```python
from build123d import *

# Parameters (mm, degrees)
F0_W           = 60
F0_H           = 20
F1_DEPTH       = 40
F3_DEPTH       = 20.001
F4_R           = 4
F5_DEPTH       = 40.001
F7_D           = 7.4
F7_DEPTH       = 30
F7_CBORE_D     = 14.25
F7_CBORE_DEPTH = 8
F7_TIP         = 2.2231842904


with BuildPart() as f1:
    # F0 (on Front) → F1 (new body)
    with BuildSketch(Plane.XZ):
        Rectangle(F0_W, F0_H)
    extrude(amount=-F1_DEPTH)

    # F2 (on face) → F3 (cut, through all)
    with BuildSketch(Plane.XY.offset(10)):
        Polygon((-30, 10.5), (-0.5, 40), (-30, 40), align=None)
        Polygon((30, 40), (0.5, 40), (30, 10.5), align=None)
    extrude(amount=-F3_DEPTH, mode=Mode.SUBTRACT)

    # F4 (on face) → F5 (cut, through all)
    with BuildSketch(Plane.XZ):
        with Locations((-20, -10)):
            Circle(F4_R)
        with Locations((20, -10)):
            Circle(F4_R)
    extrude(amount=-F5_DEPTH, mode=Mode.SUBTRACT)

    # F7
    with Locations(Plane.XY.offset(10)):
        with Locations((0, 20)):
            CounterBoreHole(F7_D / 2, F7_CBORE_D / 2, F7_CBORE_DEPTH, depth=F7_DEPTH)
            with Locations((0, 0, -(F7_DEPTH + F7_TIP / 2))):  # 118° drill point
                Cone(0, F7_D / 2, F7_TIP, mode=Mode.SUBTRACT)


solid = f1.part
```
CAD build for the part. Positions are in the model's coordinates, mm. A direction names the side the tool comes from. Coordinates: 2 decimals unless noted, no trailing zeros. Loops run counter-clockwise (first coordinate to the right, second up) from the corner with the lowest first, then second, coordinate; pieces in that order, holes last. Notation, with made-up numbers: (-9, -6) - (23, -6) arc R20 ccw to (23, 19) - close; hole circle Ø5 at (74, -31). An arc over 180 degrees is marked (long way). Return JSON: item names as keys, results as strings.
1. Probe L1, parallel to Y at x = 0, z = 8 (3 decimals); L2, parallel to Y at x = 0, z = -3.25; L3, parallel to X at y = 21, z = 0.75. List the from-to ranges inside material, lowest first. Write a range as from..to.
Result:
{"L1": "y = 0..12.875, 27.125..40", "L2": "y = 0..16.3, 23.7..40", "L3": "x = -19.5..-3.56, 3.56..19.5"}
2. Band-saw the part on D-D (x = -5). Give the cut face in (y, z).
Result:
{"outline": "(0, -10) - (35.5, -10) - (35.5, 10) - (25.08, 10) - (25.08, 2) - (14.92, 2) - (14.92, 10) - (0, 10) - close"}
3. 3-axis set-ups, long thin cutter, end or side, ignore diameter. For faces 4 (the cylindrical face through (-1.545, 13.044, 6.056)), 5 (the flat face through (27, 6, -10)): which of +Z, -Z, +X, -X, +Y, -Y reach the whole face in a straight line?
Result:
{"face 4": "+Z", "face 5": "-Z, +X, -X, +Y, -Y"}
4. Band-saw the part on A-A (z = -7.75). Give the cut face in (x, y), and give its area (3 significant figures).
Result:
{"outline": "(-30, 0) - (-23.31, 0) - (-23.31, 17.19) - (-30, 10.5) - close; (-16.69, 0) - (16.69, 0) - (16.69, 23.81) - (0.5, 40) - (-0.5, 40) - (-16.69, 23.81) - close; (23.31, 0) - (30, 0) - (30, 10.5) - (23.31, 17.19) - close; hole circle Ø7.4 at (0, 20)", "area": "1,220 mm2"}
5. Drop flat-ended pins along their axis: pin 1 (5 mm diameter, centred on y = 20, z = -3, fed in from -X); pin 2 (1 mm diameter, centred on y = 23, z = 1, fed in from -X); pin 3 (6 mm diameter, centred on x = 0, y = 20, fed in from -Z); pin 4 (10 mm diameter, centred on x = 22, y = 23, fed in from -Z). Give the stop position or say it passes through.
Result:
{"pin 1": "stops at x = -23", "pin 2": "stops at x = -18", "pin 3": "passes through", "pin 4": "stops at z = -7.35"}
6. Band-saw the part on C-C (z = -1.5). Give the cut face in (x, y).
Result:
{"outline": "(-30, 0) - (30, 0) - (30, 10.5) - (0.5, 40) - (-0.5, 40) - (-30, 10.5) - close; hole circle Ø7.4 at (0, 20)"}
7. Mould opens along Y. For faces 1 (the flat face through (-15.5, 25, 0.1)), 2 (the flat face through (0, 15, -10)), 3 (the cylindrical face through (-1.71, 16.72, -4.08)) say: released by +Y, released by -Y, zero draft, split by the parting line, or undercut.
Result:
{"face 1": "released by +Y", "face 2": "zero draft", "face 3": "undercut"}
8. Band-saw the part on B-B (y = 19). Give the cut face in (x, z), and give its area (3 significant figures).
Result:
{"outline": "(-21.5, -6.29) arc R4 cw to (-16, -10) - (-3.56, -10) - (-3.56, 2) - (-7.05, 2) - (-7.05, 10) - (-21.5, 10) - close; (3.56, -10) - (16, -10) arc R4 cw to (21.5, -6.29) - (21.5, 10) - (7.05, 10) - (7.05, 2) - (3.56, 2) - close", "area": "625 mm2"}
